Check sheet for the modelled part. Datum: model origin and axes. Units: mm. A direction names the side the tool comes from. Round coordinates to 2 decimals unless told otherwise and drop trailing zeros. Write each loop counter-clockwise with the first axis right and the second up, starting at its lowest first coordinate (ties: lowest second). Pieces come first, ordered by that corner, then holes. Notation, with made-up numbers: (32, 58.25) - (87, 58.25) arc R18 cw to (87, 84.25) - close; hole circle Ø3 at (4, 10.25). An arc over 180 degrees is marked (long way). Use one line per item in the form item = value. Start each with the question number.
1) Section check B-B (z = 0). Count the separate pieces of the cut face and the enclosed holes in it, then the cut area to 3 significant figures.
2) Section check C-C (x = 21.5). Record the boundary of the cut face in (y, z), then the cut area to 3 significant figures.
3) Section check A-A (y = 120). Record the boundary of the cut face in (x, z).
4) Gauge pin test, flat ends, axial feed: P1, Ø21, axis at y = 0, z = 0, coming from the -X side; P2, Ø4, axis at y = 84.5, z = 18.5, coming from the -X side; P3, Ø4, axis at x = 23.5, z = 17.5, coming from the +Y side. Record the tip position at first contact, or that the pin passes through.
5) Scan lines: probe 1 along Y at (x, z) = (75, 0); probe 2 along X at (y, z) = (25, -10); probe 3 along X at (y, z) = (153, 0). Record each from-to range of solid material in increasing order.
6) Draft check along X on faces 1 (the face through (-4.014, -12.69, 24.397)), 2 (the face through (-0.188, 19.56, -0.861)), 3 (the face through (67.43, -11.59, 15.12)), 4 (the face through (-3.125, 3.799, -17.108)). Enter one of: +X half, -X half, draft (parallel to the pull), parting line (faces both ways), or undercut.
7) Set-up check for faces 5 (the face through (172, 200, -19)), 6 (the face through (203.403, 198.986, 10.533)), 7 (the face through (195.976, 195.146, 7.453)): record each of +Z, -Z, +X, -X, +Y, -Y from which the full face is reachable in a straight line by a thin tool's end or side.
from build123d import *

# Parameters (mm, degrees)
SKETCH_2_R               = 19.05
SKETCH_2_R_2             = 17.4
SKETCH_2_2_R             = 19.05
SKETCH_2_2_R_2           = 17.4
CUT_EXTRUDE_1_REACH      = 293.662
SKETCH_6_R               = 17.4
CUT_EXTRUDE_2_REACH      = 309.803
SKETCH_7_R               = 17.4
CHAMFER_1_SIZE           = 2
CUT_EXTRUDE_3_DEPTH      = 289.073775273
CUT_EXTRUDE_3_DEPTH_BACK = 289.073775273
SKETCH_8_R               = 3


with BuildPart() as part:
    # Sweep 1: sweep along a path in Sketch 1
    with BuildLine(Plane.XY) as sweep_1_path:
        Line((0, 0), (133, 0))
        ThreePointArc((133, 0), (164.819805153, 13.180194847), (178, 45))
        Line((178, 45), (178, 195))
    # Sketch 2 → Sweep 1 (sweep)
    with BuildSketch(Plane(origin=(0, 0, 0), x_dir=(0, 0, -1), z_dir=(1, 0, 0))):
        Circle(SKETCH_2_R)
        Circle(SKETCH_2_R_2, mode=Mode.SUBTRACT)
    sweep(path=sweep_1_path.line)



with BuildPart() as body_2:
    # Sweep 2: sweep along a path in Sketch 1_2
    with BuildLine(Plane.XY) as sweep_2_path:
        Line((0, 0), (133, 0))
        ThreePointArc((133, 0), (164.819805153, 13.180194847), (178, 45))
        Line((178, 45), (178, 195))
    # Sketch 2_2 → Sweep 2 (sweep)
    with BuildSketch(Plane(origin=(0, 0, 0), x_dir=(0, 0, -1), z_dir=(1, 0, 0))):
        Circle(SKETCH_2_2_R)
        Circle(SKETCH_2_2_R_2, mode=Mode.SUBTRACT)
    sweep(path=sweep_2_path.line)


with BuildPart() as part_1:
    add(part.part)

    add(body_2.part)  # Revolve 1 merges body 2
    # Sketch 4 → Revolve 1 (revolve)
    with BuildSketch(Plane.XY, mode=Mode.PRIVATE) as revolve_1_sk:
        Polygon((0, 0), (0, 19.05), (-3, 27.5), (-5, 27.5), (-5, 0), align=None)
    revolve(revolve_1_sk.sketch.rotate(Axis((-5, 0, 0), (1, 0, 0)), 180), axis=Axis((-5, 0, 0), (1, 0, 0)))

    # Sketch 5 → Revolve 2 (revolve)
    with BuildSketch(Plane.XY):
        Polygon((178, 195), (178, 200), (205.5, 200), (205.5, 198), (197.05, 195), align=None)
    revolve(axis=Axis((178, 195, 0), (0, 1, 0)))

    # Sketch 6 → Cut-Extrude 1 (cut, up to next)
    with BuildSketch(Plane.ZY.offset(5), mode=Mode.PRIVATE) as cut_extrude_1_sk1:
        with Locations(Location((0, 0, 0), (0, 0, 270))):
            Circle(SKETCH_6_R)
    cut_extrude_1_tool1 = extrude(cut_extrude_1_sk1.sketch, amount=-CUT_EXTRUDE_1_REACH, mode=Mode.PRIVATE) & part_1.part
    add(cut_extrude_1_tool1.solids().sort_by_distance((-5, 0, 0))[0], mode=Mode.SUBTRACT)

    # Sketch 7 → Cut-Extrude 2 (cut, up to next)
    with BuildSketch(Plane(origin=(0, 200, 0), x_dir=(1, 0, 0), z_dir=(0, 1, 0)), mode=Mode.PRIVATE) as cut_extrude_2_sk1:
        with Locations(Location((178, 0, 0), (0, 0, 270))):
            Circle(SKETCH_7_R)
    cut_extrude_2_tool1 = extrude(cut_extrude_2_sk1.sketch, amount=-CUT_EXTRUDE_2_REACH, mode=Mode.PRIVATE) & part_1.part
    add(cut_extrude_2_tool1.solids().sort_by_distance((178, 200, 0))[0], mode=Mode.SUBTRACT)

    # Chamfer 1
    chamfer_1_edges = [part_1.edges().sort_by_distance(p)[0] for p in [
        (-5, 17.4, 0),
        (178, 200, -17.4),
    ]]
    chamfer(chamfer_1_edges, length=CHAMFER_1_SIZE)

    # Sketch 8 → Cut-Extrude 3 (cut, two sides: drawn at the far end of the back side and taken through both)
    with BuildSketch(Plane(origin=(0, 0, 0), x_dir=(0, 0, -1), z_dir=(1, 0, 0)).offset(-CUT_EXTRUDE_3_DEPTH_BACK)):
        with Locations((0, 142.5)):
            Circle(SKETCH_8_R)
    extrude(amount=CUT_EXTRUDE_3_DEPTH + CUT_EXTRUDE_3_DEPTH_BACK, mode=Mode.SUBTRACT)


solid = part_1.part
Results are:
q1.separate_pieces = 4
q1.enclosed_holes = 0
q1.area = 1,290 mm²
q2.outline = circle Ø38.1 at (0, 0); hole circle Ø34.8 at (0, 0)
q2.area = 189 mm²
q3.outline = circle Ø38.1 at (178, 0); hole circle Ø34.8 at (178, 0)
q4.P1 = 161.52
q4.P2 = 168.48
q4.P3 = 11.07
q5.probe_1 = -19.05 to -17.4, 17.4 to 19.05
q5.probe_2 = -5 to -2.8, 153.7 to 156.37, 188.76 to 190.85
q5.probe_3 = 158.95 to 160.6, 195.4 to 197.05
q6.face_1 = draft
q6.face_2 = undercut
q6.face_3 = undercut
q6.face_4 = -X half
q7.face_5 = +Z, -Z, +X, -X, +Y
q7.face_6 = +Y
q7.face_7 = none
